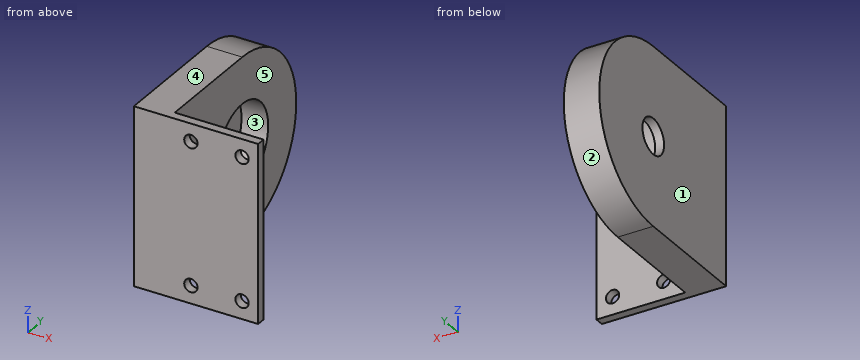
from build123d import *

# Parameters (mm, degrees)
BOSS_EXTRUDE1_DEPTH      = 6
BOSS_EXTRUDE1_DEPTH_BACK = 2
CUT_EXTRUDE1_DEPTH       = 6
SKETCH3_R                = 4
CUT_EXTRUDE2_DEPTH       = 10
SKETCH4_W                = 40
SKETCH4_H                = 2
BOSS_EXTRUDE2_DEPTH      = 20
SKETCH5_R                = 1.5
CUT_EXTRUDE3_DEPTH       = 10


with BuildPart() as part:
    # Sketch1 → Boss-Extrude1 (new, two sides: drawn at the far end of the back side and taken through both)
    with BuildSketch(Plane(origin=(0, 0, 0), x_dir=(0, 0, -1), z_dir=(1, 0, 0)).offset(-BOSS_EXTRUDE1_DEPTH_BACK)):
        with BuildLine():
            Line((-25.25, 9.083333333), (-25.25, -17.916666667))
            Line((-25.25, -17.916666667), (14.75, -17.916666667))
            Line((14.75, -17.916666667), (14.75, 9.083333333))
            ThreePointArc((14.75, 9.083333333), (-5.25, 29.083333333), (-25.25, 9.083333333))
        make_face()
    extrude(amount=BOSS_EXTRUDE1_DEPTH + BOSS_EXTRUDE1_DEPTH_BACK)

    # Sketch2 → Cut-Extrude1 (cut)
    with BuildSketch(Plane(origin=(6, 0, 0), x_dir=(0, 0, -1), z_dir=(1, 0, 0))):
        with BuildLine():
            ThreePointArc((4.35, 9.083333333), (-5.25, 18.683333333), (-14.85, 9.083333333))
            Line((-14.85, 9.083333333), (4.35, 9.083333333))
        make_face()
        with BuildLine():
            Line((4.35, 9.083333333), (-14.85, 9.083333333))
            ThreePointArc((-14.85, 9.083333333), (-5.25, -0.516666667), (4.35, 9.083333333))
        make_face()
    extrude(amount=-CUT_EXTRUDE1_DEPTH, mode=Mode.SUBTRACT)

    # Sketch3 → Cut-Extrude2 (cut)
    with BuildSketch(Plane(origin=(6, 0, 0), x_dir=(0, 0, -1), z_dir=(1, 0, 0))):
        with Locations((-5.25, 9.083333333)):
            Circle(SKETCH3_R)
    extrude(amount=-CUT_EXTRUDE2_DEPTH, mode=Mode.SUBTRACT)

    # Sketch4 → Boss-Extrude2 (add)
    with BuildSketch(Plane(origin=(6, 0, 0), x_dir=(0, 0, -1), z_dir=(1, 0, 0))):
        with Locations((-5.25, -16.916666667)):
            Rectangle(SKETCH4_W, SKETCH4_H)
    extrude(amount=BOSS_EXTRUDE2_DEPTH)

    # Sketch5 → Cut-Extrude3 (cut)
    with BuildSketch(Plane(origin=(0, -15.916666667, 0), x_dir=(1, 0, 0), z_dir=(0, 1, 0))):
        with Locations(Location((10.84792286, 10.75, 0), (0, 0, 270))):
            Circle(SKETCH5_R)
        with Locations(Location((22.368694263, 10.75, 0), (0, 0, 270))):
            Circle(SKETCH5_R)
        with Locations(Location((10.84792286, -21.25, 0), (0, 0, 270))):
            Circle(SKETCH5_R)
        with Locations(Location((22.368694263, -21.25, 0), (0, 0, 270))):
            Circle(SKETCH5_R)
    extrude(amount=-CUT_EXTRUDE3_DEPTH, mode=Mode.SUBTRACT)


solid = part.part
Geometry: final body of the model. Coordinates: model frame, mm. Face numbers are marked on the shaded views. A direction names the side the tool comes from. Give positions to 0.01 mm unless a question says otherwise; leave off trailing zeros. Loops run counter-clockwise (first coordinate to the right, second up) from the corner with the lowest first, then second, coordinate; pieces in that order, holes last. Notation, with made-up numbers: M -21,41 L 30,41 A26 cw 30,69 Z; hole C 55,72 d11. An arc over 180 degrees is marked long. Put each result on its own line as item: value.
1) Cut plane D-D, the plane y = 12.5. Return the cut outline in (x, z).
Computed values:
outline: M -2,-14.46 L 6,-14.46 L 6,-3.72 L 0,-3.72 L 0,3.17 L -2,3.17 Z; M -2,7.33 L 0,7.33 L 0,14.22 L 6,14.22 L 6,24.96 L -2,24.96 Z
2) First-contact query: P1, Ø3, axis at x = 2, y = 19, coming from the +Z side; P2, Ø5, axis at x = 10.85, z = -10.75, coming from the +Y side; P3, Ø20, axis at y = 10, z = 9, coming from the +X side. Flat tips, straight axial feed; report the tip coordinate or a pass-through.
Computed values:
P1: stops at z = 23.39
P2: stops at y = -15.92
P3: stops at x = 6
3) Mould query, pull axis Z, two halves, no side actions, for the marked faces 1, 2 and 3. Classes: released by +Z, released by -Z, zero draft, split by the parting line, or undercut.
Computed values:
face 1: zero draft
face 2: split by the parting line
face 3: undercut
4) Cut plane C-C, the plane z = -10.75. Return the cut outline in (x, y), plus the area to 3 significant figures.
Computed values:
outline: M -2,-17.92 L 9.35,-17.92 L 9.35,-15.92 L 6,-15.92 L 6,21.08 L -2,21.08 Z; M 12.35,-17.92 L 20.87,-17.92 L 20.87,-15.92 L 12.35,-15.92 Z; M 23.87,-17.92 L 26,-17.92 L 26,-15.92 L 23.87,-15.92 Z
area: 340 mm^2
5) Reachability of the marked faces 4 and 5 from +Z, -Z, +X, -X, +Y, -Y: full face, straight path, thin tool, end or side. Return the list, or none.
Computed values:
face 4: +Z, +X, -X, +Y, -Y
face 5: +Z, -Z, +X, +Y
6) Cut plane B-B, the plane z = 5.25. Return the cut outline in (x, y).
Computed values:
outline: M -2,-17.92 L 26,-17.92 L 26,-15.92 L 6,-15.92 L 6,-0.52 L 0,-0.52 L 0,5.08 L -2,5.08 Z; M -2,13.08 L 0,13.08 L 0,18.68 L 6,18.68 L 6,29.08 L -2,29.08 Z
7) Material intervals for L1, parallel to X at y = -17.1, z = -10.75; L2, parallel to Y at x = 2.35, z = 5.25; L3, parallel to Y at x = -1.1, z = 5.25, sorted ascending. Write a range as from..to.
Computed values:
L1: x = -2..9.35, 12.35..20.87, 23.87..26
L2: y = -17.92..-0.52, 18.68..29.08
L3: y = -17.92..5.08, 13.08..29.08
8) Cut plane A-A, the plane x = 1.75. Return the cut outline in (y, z), plus the area to 3 significant figures.
Computed values:
outline: M -17.92,-14.75 L 9.08,-14.75 A20 ccw 9.08,25.25 L -17.92,25.25 Z; hole C 9.08,5.25 d19.2
area: 1,420 mm^2
